from build123d import *

# Parameters (mm, degrees)
BOSS_EXTRUDE1_DEPTH             = 10
SKIZZE2_W                       = 75
SKIZZE2_H                       = 9
AUFSATZ_LINEAR_AUSTRAGEN1_DEPTH = 10
SCHNITT_LINEAR_AUSTRAGEN2_DEPTH = 10
SKIZZE4_W                       = 20
SKIZZE4_H                       = 48
AUFSATZ_LINEAR_AUSTRAGEN2_DEPTH = 3
SKIZZE5_W                       = 10
SKIZZE5_H                       = 10
SCHNITT_LINEAR_AUSTRAGEN3_DEPTH = 10


with BuildPart() as part:
    # Sketch1 → Boss-Extrude1 (new body)
    with BuildSketch(Plane.XY):
        with BuildLine():
            Line((7, 0), (0, 0))
            Line((0, 0), (0, 47.7))
            Line((0, 47.7), (0, 55))
            ThreePointArc((0, 55), (8.786796564, 76.213203436), (30, 85))
            Line((30, 85), (32, 85))
            Line((32, 85), (32, 65))
            Line((32, 65), (22, 65))
            ThreePointArc((22, 65), (11.393398282, 60.606601718), (7, 50))
            Line((7, 50), (7, 0))
        make_face()
    extrude(amount=BOSS_EXTRUDE1_DEPTH)

    # Skizze2 → Aufsatz-Linear austragen1 (add)
    with BuildSketch(Plane(origin=(0, 0, 0), x_dir=(-1, 0, 0), z_dir=(0, 0, -1))):
        with Locations((-37.5, 43.5)):
            Rectangle(SKIZZE2_W, SKIZZE2_H)
    extrude(amount=AUFSATZ_LINEAR_AUSTRAGEN1_DEPTH)

    # Skizze3 → Schnitt-Linear austragen2 (cut)
    with BuildSketch(Plane(origin=(0, 0, -10), x_dir=(-1, 0, 0), z_dir=(0, 0, -1))):
        Polygon((-3.370852377, 43.5254), (-1.647110898, 43.5254), (0, 39), (-5.017963275, 39), align=None)
        Polygon((-9.670852377, 43.5254), (-7.947110898, 43.5254), (-6.3, 39), (-11.317963275, 39), align=None)
        Polygon((-15.970852377, 43.5254), (-14.247110898, 43.5254), (-12.6, 39), (-17.617963275, 39), align=None)
        Polygon((-22.270852377, 43.5254), (-20.547110898, 43.5254), (-18.9, 39), (-23.917963275, 39), align=None)
        Polygon((-28.570852377, 43.5254), (-26.847110898, 43.5254), (-25.2, 39), (-30.217963275, 39), align=None)
        Polygon((-34.870852377, 43.5254), (-33.147110898, 43.5254), (-31.5, 39), (-36.517963275, 39), align=None)
        Polygon((-41.170852377, 43.5254), (-39.447110898, 43.5254), (-37.8, 39), (-42.817963275, 39), align=None)
        Polygon((-47.470852377, 43.5254), (-45.747110898, 43.5254), (-44.1, 39), (-49.117963275, 39), align=None)
        Polygon((-53.770852377, 43.5254), (-52.047110898, 43.5254), (-50.4, 39), (-55.417963275, 39), align=None)
        Polygon((-60.070852377, 43.5254), (-58.347110898, 43.5254), (-56.7, 39), (-61.717963275, 39), align=None)
        Polygon((-66.370852377, 43.5254), (-64.647110898, 43.5254), (-63, 39), (-68.017963275, 39), align=None)
        Polygon((-72.670852377, 43.5254), (-70.947110898, 43.5254), (-69.3, 39), (-74.317963275, 39), align=None)
    extrude(amount=-SCHNITT_LINEAR_AUSTRAGEN2_DEPTH, mode=Mode.SUBTRACT)

    # Skizze4 → Aufsatz-Linear austragen2 (add)
    with BuildSketch(Plane.ZY):
        with Locations((0, 24)):
            Rectangle(SKIZZE4_W, SKIZZE4_H)
    extrude(amount=-AUFSATZ_LINEAR_AUSTRAGEN2_DEPTH)

    # Skizze5 → Schnitt-Linear austragen3 (cut)
    with BuildSketch(Plane(origin=(3, 0, 0), x_dir=(0, 0, -1), z_dir=(1, 0, 0))):
        with Locations((5, 5)):
            Rectangle(SKIZZE5_W, SKIZZE5_H)
    extrude(amount=-SCHNITT_LINEAR_AUSTRAGEN3_DEPTH, mode=Mode.SUBTRACT)


solid = part.part
Could you check a few things on this model? Use its own coordinates, in mm. A direction names the side the tool comes from. Give positions to 0.01 mm unless a question says otherwise; leave off trailing zeros. Order: outer loops, then holes, each group sorted by start corner. A loop starts at its lowest first (then second) coordinate and runs counter-clockwise, first axis right, second up.
1. Suppose I cut it at A-A (z = 8.25). Write out the boundary of the cut face in (x, y), plus the area to 3 significant figures.
Answers below:
outline: (0, 0) - (7, 0) - (7, 50) arc R15 cw to (22, 65) - (32, 65) - (32, 85) - (30, 85) arc R30 ccw to (0, 55) - close
area: 950 mm2
2. I need wall thicknesses on L1, parallel to Z at x = 10, y = 66.5; L2, parallel to X at y = 17.5, z = 9.25; L3, parallel to Y at x = 31, z = -2.75. Which ranges of each line are inside material? Lowest first, please.
Answers below:
L1: z = 0 to 10
L2: x = 0 to 7
L3: y = 39 to 48
3. Suppose I cut it at B-B (y = 30.5). Write out the boundary of the cut face in (x, z), plus the area to 3 significant figures.
Answers below:
outline: (0, -10) - (3, -10) - (3, 0) - (7, 0) - (7, 10) - (0, 10) - close
area: 100 mm2
4. For pin 1 (12 mm diameter, centred on x = 52, z = 4, fed in from +Y); pin 2 (1 mm diameter, centred on x = 69, z = -4, fed in from -Y); pin 3 (0.9 mm diameter, centred on x = 59, z = -7.5, fed in from -Y), each with a flat end and sliding along its axis, tell me the tip position at first contact or that it passes through.
Answers below:
pin 1: stops at y = 48
pin 2: stops at y = 39
pin 3: stops at y = 43.53
5. Thinking about a two-plate mould opening in X: for faces 4 (the cylindrical face through (8.555, 75.979, 4.93)), 5 (the cylindrical face through (11.51, 60.72, 4.93)), 6 (the flat face through (29.406, 41.231, -5.07)), 7 (the flat face through (3, 0, 5)), which applies, +X half, -X half, draft (parallel to the pull), parting line (faces both ways), or undercut?
Answers below:
face 4: -X half
face 5: +X half
face 6: undercut
face 7: draft
6. Which directions (+Z, -Z, +X, -X, +Y, -Y) give clear straight access to the entire face, cutting with the end or side of a thin tool? Please do faces 1 (the flat face through (16, 71, 0)), 2 (the flat face through (16.806, 41.231, -5.07)), 3 (the flat face through (2, 10, -5)).
Answers below:
face 1: -Z, +X, -X, +Y
face 2: +Z, -Z, -Y
face 3: -Z, +X, -X, -Y
